Verification items for the finished model (mm, model axes). Face numbers are marked on the shaded views. Coordinates: 2 decimals unless noted, no trailing zeros. Loops run counter-clockwise (first coordinate to the right, second up) from the corner with the lowest first, then second, coordinate; pieces in that order, holes last. Notation, with made-up numbers: (9, 34.25) -> (35, 34.25) arc R21 cw to (35, 59.25) -> close; hole circle Ø4 at (44, 18). An arc over 180 degrees is marked (long way). Use CSV: the item, a comma, the result in double quotes. Start each with the question number.
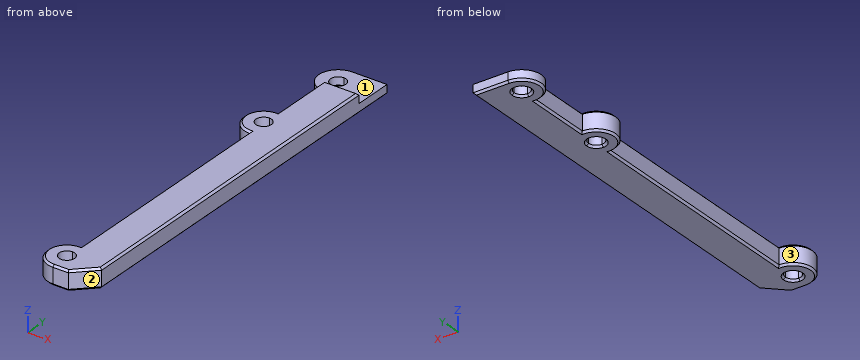
```python
from build123d import *

# Parameters (mm, degrees)
F1_DEPTH = 5
F3_DEPTH = 2.5
F4_SIZE  = 5
F5_SIZE  = 0.5


with BuildPart() as f1:
    # F0 (on Top) → F1 (new body)
    with BuildSketch(Plane.XY):
        with BuildLine():
            Line((-9, 0), (0, 0))
            Line((0, 0), (0, 106.5))
            Line((0, 106.5), (-9, 106.5))
            Line((-9, 106.5), (-9, 103.5))
            ThreePointArc((-9, 103.5), (-7.5857864376, 102.9142135624), (-7, 101.5))
            ThreePointArc((-7, 101.5), (-7.5857864376, 100.0857864376), (-9, 99.5))
            Line((-9, 99.5), (-9, 96.5))
            Line((-9, 96.5), (-9, 80))
            Line((-9, 80), (-9, 77))
            ThreePointArc((-9, 77), (-7.5857864376, 76.4142135624), (-7, 75))
            ThreePointArc((-7, 75), (-7.5857864376, 73.5857864376), (-9, 73))
            Line((-9, 73), (-9, 70))
            Line((-9, 70), (-9, 10))
            Line((-9, 10), (-9, 7))
            ThreePointArc((-9, 7), (-7.5857864376, 6.4142135624), (-7, 5))
            ThreePointArc((-7, 5), (-7.5857864376, 3.5857864376), (-9, 3))
            Line((-9, 3), (-9, 0))
        make_face()
        with BuildLine():
            ThreePointArc((-9, 10), (-14, 5), (-9, 0))
            Line((-9, 0), (-9, 3))
            ThreePointArc((-9, 3), (-11, 5), (-9, 7))
            Line((-9, 7), (-9, 10))
        make_face()
        with BuildLine():
            Line((-9, 103.5), (-9, 106.5))
            ThreePointArc((-9, 106.5), (-14, 101.5), (-9, 96.5))
            Line((-9, 96.5), (-9, 99.5))
            ThreePointArc((-9, 99.5), (-11, 101.5), (-9, 103.5))
        make_face()
        with BuildLine():
            ThreePointArc((-9, 80), (-14, 75), (-9, 70))
            Line((-9, 70), (-9, 73))
            ThreePointArc((-9, 73), (-11, 75), (-9, 77))
            Line((-9, 77), (-9, 80))
        make_face()
    extrude(amount=F1_DEPTH)

    # F2 (on face) → F3 (cut)
    with BuildSketch(Plane.XY.offset(5)):
        with BuildLine():
            ThreePointArc((-9, 106.5), (-14, 101.5), (-9, 96.5))
            Line((-9, 96.5), (0, 96.5))
            Line((0, 96.5), (0, 106.5))
            Line((0, 106.5), (-9, 106.5))
        make_face()
    extrude(amount=-F3_DEPTH, mode=Mode.SUBTRACT)

    # F4
    f4_edges = [f1.edges().sort_by_distance(p)[0] for p in [
        (0, 0, 2.5),
    ]]
    chamfer(f4_edges, length=F4_SIZE)

    # F5
    f5_edges = [f1.edges().sort_by_distance(p)[0] for p in [
        (-7, 0, 0),
        (-2.5, 2.5, 0),
        (-14, 5, 0),
        (0, 55.75, 0),
        (-9, 40, 0),
        (-4.5, 106.5, 0),
        (-14, 75, 0),
        (-14, 101.5, 0),
        (-9, 88.25, 0),
        (-9, 77, 0),
        (-9, 103.5, 0),
        (-11, 5, 0),
        (-4.5, 96.5, 5),
        (0, 50.75, 5),
        (-9, 88.25, 5),
        (-14, 75, 5),
        (-2.5, 2.5, 5),
        (-7, 0, 5),
        (-14, 5, 5),
        (-9, 40, 5),
    ]]
    chamfer(f5_edges, length=F5_SIZE)


solid = f1.part
```
1. Scan lines: line 1 (Y direction, x = -9.5, z = 2.95); line 2 (Y direction, x = -12.5, z = 2); line 3 (X direction, y = 38, z = 3.1). Record each from-to range of solid material in increasing order.
2. Release check for a two-part mould opening along Y. For the marked faces 1, 2 and 3 record: released by +Y, released by -Y, zero draft, split by the parting line, or undercut.
3. Cross-section at B-B, the plane y = 50. Record the boundary of the cut face in (x, z).
4. Cross-section at C-C, the plane x = -1.75. Record the boundary of the cut face in (y, z).
5. Depth check by flat-ended pin: pin 1 (5 mm diameter, centred on x = -5.5, y = 101, fed in from +Z); pin 2 (2 mm diameter, centred on y = 46, z = 2, fed in from -X); pin 3 (0.6 mm diameter, centred on x = -4, z = 3, fed in from +Y). Enter the tip coordinate at first touch or a pass-through.
6. Cross-section at A-A, the plane z = 3.4. Record the boundary of the cut face in (x, y), plus the area to 3 significant figures.
Solution:
1,line 1,"y = 0.03 to 3.06, 6.94 to 9.97, 70.03 to 73.06, 76.94 to 79.97"
1,line 2,"y = 1.43 to 8.57, 71.43 to 78.57, 97.93 to 105.07"
1,line 3,"x = -9 to 0"
2,face 1,"zero draft"
2,face 2,"released by -Y"
2,face 3,"undercut"
3,outline,"(-9, 0.5) -> (-8.5, 0) -> (-0.5, 0) -> (0, 0.5) -> (0, 4.5) -> (-0.5, 5) -> (-8.5, 5) -> (-9, 4.5) -> close"
4,outline,"(3.25, 0.5) -> (3.96, 0) -> (106, 0) -> (106.5, 0.5) -> (106.5, 2.5) -> (96.5, 2.5) -> (96.5, 4.5) -> (96, 5) -> (3.96, 5) -> (3.25, 4.5) -> close"
5,pin 1,"stops at z = 2.5"
5,pin 2,"stops at x = -9"
5,pin 3,"stops at y = 96.5"
6,outline,"(-9, 0) -> (-5, 0) -> (0, 5) -> (0, 96.5) -> (-9, 96.5) -> (-9, 80) arc R5 ccw to (-9, 70) -> (-9, 10) arc R5 ccw to start; hole circle Ø4 at (-9, 5); hole circle Ø4 at (-9, 75)"
6,area,"909 mm2"
